Read the model definition and answer for the solid it produces. Units are mm, in the model's axes. Give positions to 0.01 mm unless a question says otherwise; leave off trailing zeros. Write each loop counter-clockwise with the first axis right and the second up, starting at its lowest first coordinate (ties: lowest second). Pieces come first, ordered by that corner, then holes. Notation, with made-up numbers: (25, 22) -> (57, 22) arc R5 ccw to (57, 27) -> close; hole circle Ø2 at (48, 9). An arc over 180 degrees is marked (long way). Answer as CSV lines item,"result". Start each with the question number.
1. The part is cut by section B-B, the plane x = 39.5. Determine the outline of the cut face in (y, z).
2. Given pin 1 (3 mm diameter, centred on x = 48.5, z = 35, fed in from -Y), flat-ended and moving along its own axis, determine where the tip first touches the part or whether it passes through.
3. The part is cut by section A-A, the plane y = 1.2. Give the number of separate pieces and of enclosed holes in the cut face, and give its area (3 significant figures).
4. Find the intervals of material crossed by line 1 (Z direction, x = 0, y = 1.2); line 2 (X direction, y = 0.6, z = 15.5); line 3 (X direction, y = 0.2, z = 17), in increasing order.
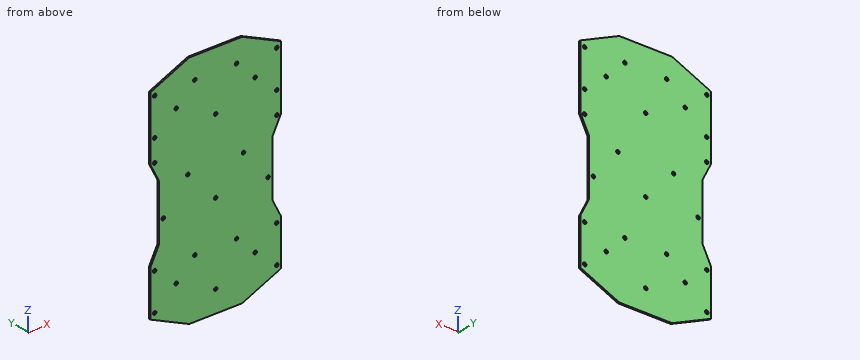
Autodesk Inventor part; units mm, degrees
ref_plane "YZ Plane" through (0, 0, 0) normal (1, 0, 0) x (0, 1, 0)
ref_plane "XZ Plane" through (0, 0, 0) normal (0, 1, 0) x (-1, 0, 0)
ref_plane "XY Plane" through (0, 0, 0) normal (0, 0, 1) x (1, 0, 0)
sketch "Sketch1" plane through (0, 0, 0) normal (0, 1, 0) x (-1, 0, 0)
  circle A0 centre (24.1, 110.65) radius 0.25
  circle A1 centre (-70.5, 110.65) radius 0.25
  circle A2 centre (-45.6, 89.15) radius 0.25
  circle A3 centre (0, 67.65) radius 0.25
  circle A4 centre (70.5, 42.15) radius 0.25
  circle A5 centre (32.15, 17.15) radius 0.25
  circle A6 centre (60.5, -17.65) radius 0.25
  circle A7 centre (-60.5, -17.65) radius 0.25
  circle A8 centre (24.1, -67.65) radius 0.25
  circle A9 centre (-70.5, -67.65) radius 0.25
  circle A10 centre (-45.6, -89.15) radius 0.25
  circle A11 centre (0, -110.65) radius 0.25
  circle A12 centre (-70.5, -110.65) radius 0.25
  circle A13 centre (70.5, -110.65) radius 0.25
  circle A14 centre (45.6, -89.15) radius 0.25
  circle A15 centre (-24.1, -67.65) radius 0.25
  circle A16 centre (70.5, -67.65) radius 0.25
  circle A17 centre (0, -17.65) radius 0.25
  circle A18 centre (-32.15, 17.15) radius 0.25
  circle A19 centre (-70.5, 42.15) radius 0.25
  circle A20 centre (-70.5, 67.65) radius 0.25
  circle A21 centre (70.5, 67.65) radius 0.25
  circle A22 centre (45.6, 89.15) radius 0.25
  circle A23 centre (-24.1, 110.65) radius 0.25
  circle A24 centre (70.5, 110.65) radius 0.25
  line L0 (75.5, -115.65) -> (75.5, -62.65)
  line L1 (75.5, -62.65) -> (65.5, -42.65)
  line L2 (65.5, -42.65) -> (65.5, 22.15)
  line L3 (65.5, 22.15) -> (75.5, 42.15)
  line L4 (75.5, 42.15) -> (75.5, 115.65)
  line L5 (75.5, 115.65) -> (30.5, 135.65)
  line L6 (30.5, 135.65) -> (-30.5, 135.65)
  line L7 (-30.5, 135.65) -> (-75.5, 115.65)
  line L8 (-75.5, 115.65) -> (-75.5, 42.15)
  line L9 (-75.5, 42.15) -> (-65.5, 22.15)
  line L10 (-65.5, 22.15) -> (-65.5, -42.65)
  line L11 (-65.5, -42.65) -> (-75.5, -62.65)
  line L12 (-75.5, -62.65) -> (-75.5, -115.65)
  line L13 (-75.5, -115.65) -> (-30.5, -135.65)
  line L14 (-30.5, -135.65) -> (30.5, -135.65)
  line L15 (30.5, -135.65) -> (75.5, -115.65)
  circle A25 centre (0, -110.65) radius 2
  circle A26 centre (70.5, -110.65) radius 2
  circle A27 centre (-70.5, -110.65) radius 2
  circle A28 centre (45.6, -89.15) radius 2
  circle A29 centre (-45.6, -89.15) radius 2
  circle A30 centre (70.5, -67.65) radius 2
  circle A31 centre (24.1, -67.65) radius 2
  circle A32 centre (-24.1, -67.65) radius 2
  circle A33 centre (-70.5, -67.65) radius 2
  circle A34 centre (60.5, -17.65) radius 2
  circle A35 centre (0, -17.65) radius 2
  circle A36 centre (-32.15, 17.15) radius 2
  circle A37 centre (-60.5, -17.65) radius 2
  circle A38 centre (32.15, 17.15) radius 2
  circle A39 centre (70.5, 42.15) radius 2
  circle A40 centre (-70.5, 42.15) radius 2
  circle A41 centre (-70.5, 67.65) radius 2
  circle A42 centre (0, 67.65) radius 2
  circle A43 centre (70.5, 67.65) radius 2
  circle A44 centre (45.6, 89.15) radius 2
  circle A45 centre (-45.6, 89.15) radius 2
  circle A46 centre (-70.5, 110.65) radius 2
  circle A47 centre (-24.1, 110.65) radius 2
  circle A48 centre (24.1, 110.65) radius 2
  circle A49 centre (70.5, 110.65) radius 2
  point P0 (0, 0)
  point P1 (0, 0)
  dimension "d0" = 4
  dimension "d1" = 4
  dimension "d2" = 4
  dimension "d3" = 4
  dimension "d4" = 4
  dimension "d5" = 4
  dimension "d6" = 4
  dimension "d7" = 4
  dimension "d8" = 4
  dimension "d9" = 4
  dimension "d10" = 4
  dimension "d11" = 4
  dimension "d12" = 4
  dimension "d13" = 4
  dimension "d14" = 4
  dimension "d15" = 4
  dimension "d16" = 4
  dimension "d17" = 4
  dimension "d18" = 4
  dimension "d19" = 4
  dimension "d20" = 4
  dimension "d21" = 4
  dimension "d22" = 4
  dimension "d23" = 4
  dimension "d24" = 4
extrude "Extrusion1" add sketch "Sketch1" along normal blind 2 contours L15 L14 L13 L12 L11 L10 L9 L8 L7 L6 L5 L4 L3 L2 L1 L0
properties part number "podvozek"
Results found:
1,outline,"(0, -131.65) -> (2, -131.65) -> (2, 131.65) -> (0, 131.65) -> close"
2,pin 1,"stops at y = 0"
3,separate pieces,"1"
3,enclosed holes,"25"
3,area,"37,200 mm²"
4,line 1,"z = -135.65 to -112.65, -108.65 to -19.65, -15.65 to 65.65, 69.65 to 135.65"
4,line 2,"x = -65.5 to -33.28, -31.02 to 31.02, 33.28 to 65.5"
4,line 3,"x = -65.5 to -34.14, -30.16 to 30.16, 34.14 to 65.5"
